Verification items for the finished model (mm, model axes). A direction names the side the tool comes from. Coordinates: 2 decimals unless noted, no trailing zeros. Write each loop counter-clockwise with the first axis right and the second up, starting at its lowest first coordinate (ties: lowest second). Pieces come first, ordered by that corner, then holes.
```python
from build123d import *

# Parameters (mm, degrees)
CROQUIS1_R              = 1.5
CROQUIS1_R_2            = 5
SALIENTE_EXTRUIR2_DEPTH = 3.5


with BuildPart() as part:
    # Croquis1 → Saliente-Extruir2 (new body)
    with BuildSketch(Plane(origin=(0, 0, 0), x_dir=(1, 0, 0), z_dir=(0, 1, 0))):
        with BuildLine():
            Line((1.47572532, 11.484579709), (1.47572532, 3.695762793))
            ThreePointArc((1.47572532, 3.695762793), (0.818994747, 2.110274939), (-0.766493108, 1.453544366))
            Line((-0.766493108, 1.453544366), (-23.52427468, 1.453544366))
            ThreePointArc((-23.52427468, 1.453544366), (-28.52427468, -3.546455634), (-23.52427468, -8.546455634))
            Line((-23.52427468, -8.546455634), (-0.766493108, -8.546455634))
            ThreePointArc((-0.766493108, -8.546455634), (0.818994747, -9.203186206), (1.47572532, -10.788674061))
            Line((1.47572532, -10.788674061), (1.47572532, -18.577490976))
            Line((1.47572532, -18.577490976), (1.47572532, -33.546455634))
            ThreePointArc((1.47572532, -33.546455634), (6.47572532, -38.546455634), (11.47572532, -33.546455634))
            Line((11.47572532, -33.546455634), (11.47572532, -10.788674061))
            Line((11.47572532, -10.788674061), (11.47572532, -10.748363891))
            ThreePointArc((11.47572532, -10.748363891), (12.133603326, -9.190173106), (13.697697252, -8.546455634))
            Line((13.697697252, -8.546455634), (36.47572532, -8.546455634))
            ThreePointArc((36.47572532, -8.546455634), (41.47572532, -3.546455634), (36.47572532, 1.453544366))
            Line((36.47572532, 1.453544366), (13.697697252, 1.453544366))
            ThreePointArc((13.697697252, 1.453544366), (12.133603326, 2.097261838), (11.47572532, 3.655452623))
            Line((11.47572532, 3.655452623), (11.47572532, 3.695762793))
            Line((11.47572532, 3.695762793), (11.47572532, 26.453544366))
            ThreePointArc((11.47572532, 26.453544366), (6.47572532, 31.453544366), (1.47572532, 26.453544366))
            Line((1.47572532, 26.453544366), (1.47572532, 11.484579709))
        make_face()
        with Locations(Location((-1.52427468, -3.546455634, 0), (0, 0, 270))):
            Circle(CROQUIS1_R, mode=Mode.SUBTRACT)
        with Locations(Location((6.47572532, -28.546455634, 0), (0, 0, 270))):
            Circle(CROQUIS1_R, mode=Mode.SUBTRACT)
        with Locations(Location((6.47572532, -12.546455634, 0), (0, 0, 270))):
            Circle(CROQUIS1_R, mode=Mode.SUBTRACT)
        with Locations(Location((-18.52427468, -3.546455634, 0), (0, 0, 270))):
            Circle(CROQUIS1_R, mode=Mode.SUBTRACT)
        with Locations(Location((6.47572532, -3.546455634, 0), (0, 0, 270))):
            Circle(CROQUIS1_R_2, mode=Mode.SUBTRACT)
        with Locations(Location((14.47572532, -3.546455634, 0), (0, 0, 270))):
            Circle(CROQUIS1_R, mode=Mode.SUBTRACT)
        with Locations(Location((6.47572532, 5.453544366, 0), (0, 0, 270))):
            Circle(CROQUIS1_R, mode=Mode.SUBTRACT)
        with Locations(Location((31.47572532, -3.546455634, 0), (0, 0, 270))):
            Circle(CROQUIS1_R, mode=Mode.SUBTRACT)
        with Locations(Location((6.47572532, 21.453544366, 0), (0, 0, 270))):
            Circle(CROQUIS1_R, mode=Mode.SUBTRACT)
    extrude(amount=SALIENTE_EXTRUIR2_DEPTH)


solid = part.part
```
1. Draft check along Z on faces 1 (the cylindrical face through (6.542, 1.726, -22.952)), 2 (the flat face through (11.476, 2, 22)), 3 (the cylindrical face through (6.586, 1.726, -31.452)). Enter one of: pulls with the +Z half, pulls with the -Z half, needs draft (parallel to the pull), parting line crosses it, or undercut.
2. Sectioned sample at B-B, the plane y = 2.9. Give the number of separate pieces and of enclosed holes in the cut face, and give its area (3 significant figures).
3. Sectioned sample at A-A, the plane z = 1. Record the boundary of the cut face in (x, y).
4. Material ranges on L1, parallel to X at y = 2.1, z = 20; L2, parallel to Z at x = 24.5, y = 3.25; L3, parallel to Z at x = -0.5, y = 3.05, recorded low to high.
5. Sectioned sample at D-D, the plane x = -22. Record the boundary of the cut face in (y, z).
6. Sectioned sample at C-C, the plane z = -8. Record the boundary of the cut face in (x, y), and give its area (3 significant figures).
7. Tool access check on faces 4 (the flat face through (-12, 2, 8.546)), 5 (the cylindrical face through (5.56, 1.73, 11.36)), 6 (the flat face through (-12, 2, -1.454)), 7 (the flat face through (6, 3.5, 9)), 8 (the flat face through (25, 2, -1.454)). Record the directions out of +Z, -Z, +X, -X, +Y, -Y that give a thin tool (end or side, any length) a straight path to the whole face; none if there is none.
8. Gauge pin test, flat ends, axial feed: P1, Ø1.8, axis at y = 2, z = 16.5, coming from the -X side; P2, Ø2, axis at x = 15.5, y = 2.5, coming from the +Z side; P3, Ø2, axis at y = 2, z = 0.5, coming from the -X side; P4, Ø2.5, axis at x = 6.48, z = 28.55, coming from the -Y side. Record the tip position at first contact, or that the pin passes through.
Outcome:
1. face 1: undercut
1. face 2: needs draft
1. face 3: pulls with the -Z half
2. separate pieces: 1
2. enclosed holes: 9
2. area: 1,130 mm2
3. outline: (-27.83, 0) - (2.17, 0) - (2.17, 3.5) - (-27.83, 3.5) - close; (10.78, 0) - (40.78, 0) - (40.78, 3.5) - (10.78, 3.5) - close
4. L1: x = 1.48 to 11.48
4. L2: z = -1.45 to 8.55
4. L3: z = -1.47 to 2.45, 4.64 to 8.56
5. outline: (0, -1.45) - (3.5, -1.45) - (3.5, 8.55) - (0, 8.55) - close
6. outline: (1.48, 0) - (11.48, 0) - (11.48, 3.5) - (1.48, 3.5) - close
6. area: 35.0 mm2
7. face 4: +Z, -X, +Y, -Y
7. face 5: +Y, -Y
7. face 6: -Z, -X, +Y, -Y
7. face 7: +Z, -Z, +X, -X, +Y
7. face 8: -Z, +X, +Y, -Y
8. P1: stops at x = 1.48
8. P2: stops at z = 8.55
8. P3: stops at x = -28.09
8. P4: passes through
